```python
from build123d import *

# Parameters (mm, degrees)
SKETCH1_W          = 101.6
SKETCH1_H          = 88.4936
SKETCH1_R          = 31.7627
EXTRUDE1_DEPTH     = 75.9968
CUT_EXTRUDE1_DEPTH = 102.6
SKETCH3_R          = 33.401
CUT_EXTRUDE2_DEPTH = 44.2468
FILLET1_R          = 0.762
HOLE1_D            = 12.7
HOLE1_DEPTH        = 88.4936


with BuildPart() as part:
    # Sketch1 → Extrude1 (new body)
    with BuildSketch(Plane.XY):
        with Locations((50.8, 44.2468)):
            Rectangle(SKETCH1_W, SKETCH1_H)
        with Locations((50.8, 45.0088)):
            Circle(SKETCH1_R, mode=Mode.SUBTRACT)
    extrude(amount=-EXTRUDE1_DEPTH)

    # Sketch2 → Cut-Extrude1 (cut, through all)
    with BuildSketch(Plane(origin=(101.6, 0, 0), x_dir=(0, 0, -1), z_dir=(1, 0, 0))):
        Polygon((0, 88.4936), (44.2468, 88.4936), (0, 7.874), align=None)
    extrude(amount=-CUT_EXTRUDE1_DEPTH, mode=Mode.SUBTRACT)

    # Sketch3 → Cut-Extrude2 (cut)
    with BuildSketch(Plane(origin=(0, 0, 0), x_dir=(-1, 0, 0), z_dir=(0, 0, -1))):
        with Locations(Location((-50.8, 45.0088, 0), (0, 0, 180))):  # turned: the seam where the file's is
            Circle(SKETCH3_R)
    extrude(amount=CUT_EXTRUDE2_DEPTH, mode=Mode.SUBTRACT)

    # Fillet1
    fillet1_edges = [part.edges().sort_by_distance(p)[0] for p in [
        (17.399, 45.0088, -44.2468),
    ]]
    fillet(fillet1_edges, radius=FILLET1_R)

    # Hole1
    with Locations(Plane(origin=(0, 88.4936, 0), x_dir=(-1, 0, 0), z_dir=(0, 1, 0))):
        with Locations((-9.9822, -59.9948), (-91.0082, -59.9948)):
            Hole(HOLE1_D / 2, depth=HOLE1_DEPTH)

    # Sketch6 → Cut-Revolve1 (revolve, cut)
    with BuildSketch(Plane(origin=(0, 45.0088, 0), x_dir=(-1, 0, 0), z_dir=(0, 1, 0)), mode=Mode.PRIVATE) as cut_revolve1_sk:
        Polygon((-17.399, -41.3258), (-17.399, -42.0878), (-17.018, -41.7068), align=None)
        Polygon((-19.0373, -75.2475), (-19.0373, -75.9968), (-18.288, -75.9968), align=None)
    revolve(cut_revolve1_sk.sketch.rotate(Axis((50.8, 45.0088, 17.508123997), (0, 0, -1)), 180), axis=Axis((50.8, 45.0088, 17.508123997), (0, 0, -1)), mode=Mode.SUBTRACT)  # turned: the seam where the file's is


solid = part.part
```
The listing builds one solid part. Answer for the finished solid, in the listing's coordinates (mm). A direction names the side the tool comes from. Round coordinates to 2 decimals unless told otherwise and drop trailing zeros. Loops run counter-clockwise (first coordinate to the right, second up) from the corner with the lowest first, then second, coordinate; pieces in that order, holes last. Notation, with made-up numbers: (65.5, 79.25) - (115.5, 79.25) arc R32 ccw to (115.5, 117.25) - close; hole circle Ø6 at (73, 52). An arc over 180 degrees is marked (long way). Return JSON: item names as keys, results as strings. Group by question number.
1. The part is cut by section B-B on z = -39. Determine the outline of the cut face in (x, y).
2. Consider probe 1 along Y at (x, z) = (51.5, -48); probe 2 along X at (y, z) = (45.5, -40); probe 3 along X at (y, z) = (45, -73). Determine where each line is inside the solid, lowest interval first.
3. The part is cut by section C-C on y = 65. State how many separate pieces and enclosed holes the cut face has, then the cut area to 3 significant figures.
4. The part is cut by section A-A on x = 50.8. Determine the outline of the cut face in (y, z), then the cut area to 3 significant figures.
5. Each of these flat-tipped pins is pushed along its axis until it touches: P1, Ø5, axis at x = 31, z = -38, coming from the +Y side; P2, Ø20.5, axis at x = 91.01, z = -59.99, coming from the -Y side; P3, Ø8, axis at y = 64, z = -23, coming from the -X side. Where does it stop, or does it pass through?
6. Which of the six approach directions +Z, -Z, +X, -X, +Y, -Y give full straight-line access (tool end or side, diameter ignored) to faces 1 (the cylindrical face through (17.43, 43.54, -42.78)), 2 (the flat face through (50, 0, -37))?
7. The part is cut by section D-D on z = -29. Determine the outline of the cut face in (x, y).
8. The mould has two halves that part along X. Classify faces 3 (the flat face through (101.6, 34, -46)), 4 (the flat face through (82, 52, -44.247)), 5 (the flat face through (0, 34, -46)): pulls with the +X half, pulls with the -X half, needs draft (parallel to the pull), parting line crosses it, or undercut.
Resolved:
{
 "1": {"outline": "(0, 0) - (101.6, 0) - (101.6, 78.93) - (0, 78.93) - close; hole circle Ø66.8 at (50.8, 45.01)"},
 "2": {"probe 1": "y = 0 to 13.25, 76.76 to 88.49", "probe 2": "x = 0 to 17.4, 84.2 to 101.6", "probe 3": "x = 0 to 19.04, 82.56 to 101.6"},
 "3": {"separate pieces": "2", "enclosed holes": "2", "area": "2,020 mm²"},
 "4": {"outline": "(0, -76) - (12.5, -76) - (13.25, -75.25) - (13.25, -44.25) - (12.37, -44.25) arc R0.76 cw to (11.61, -43.48) - (11.61, -42.09) - (11.23, -41.71) - (11.61, -41.33) - (11.61, -2.05) - (7.87, 0) - (0, 0) - close; (76.77, -75.25) - (77.52, -76) - (88.49, -76) - (88.49, -44.25) - (78.41, -38.71) - (78.41, -41.33) - (78.79, -41.71) - (78.41, -42.09) - (78.41, -43.48) arc R0.76 cw to (77.65, -44.25) - (76.77, -44.25) - close", "area": "1,330 mm²"},
 "5": {"P1": "stops at y = 81.67", "P2": "stops at y = 0", "P3": "passes through"},
 "6": {"face 1": "+Z", "face 2": "+Z, -Z, +X, -X, -Y"},
 "7": {"outline": "(0, 0) - (101.6, 0) - (101.6, 60.71) - (80.28, 60.71) arc R33.4 cw (long way) to (21.32, 60.71) - (0, 60.71) - close"},
 "8": {"face 3": "pulls with the +X half", "face 4": "undercut", "face 5": "pulls with the -X half"}
}
